The listing builds one solid part. Answer for the finished solid, in the listing's coordinates (mm). Face numbers are marked on the shaded views. Coordinates: 2 decimals unless noted, no trailing zeros. Loops run counter-clockwise (first coordinate to the right, second up) from the corner with the lowest first, then second, coordinate; pieces in that order, holes last. Notation, with made-up numbers: M 57,5.5 L 91,5.5 A15 cw 91,21.5 Z; hole C -19,17 d6. An arc over 180 degrees is marked long. Answer as CSV lines item,"result". Start each with the question number.
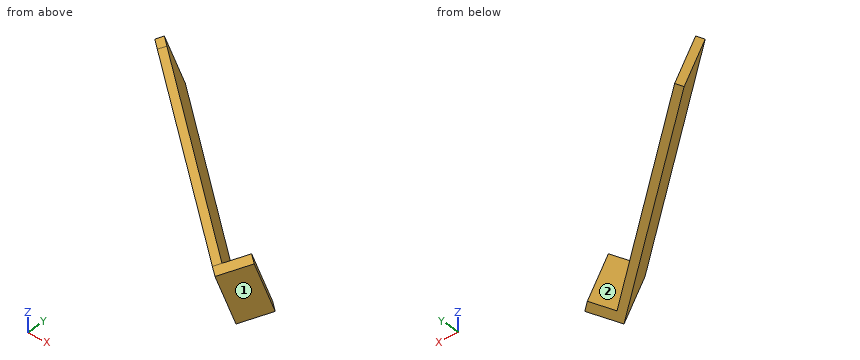
```python
from build123d import *

# Parameters (mm, degrees)
SALIENTE_EXTRUIR1_START = 3.1
SALIENTE_EXTRUIR1_DEPTH = 1
SALIENTE_EXTRUIR2_START = -1
CROQUIS4_W              = 1.301297423
CROQUIS4_H              = 8.40000117
SALIENTE_EXTRUIR2_DEPTH = 4.1


with BuildPart() as part:
    # Croquis3 → Saliente-Extruir1 (new body)
    with BuildSketch(Plane(origin=(-33.880247059, -37.627827516, -15.480136045), x_dir=(-0.768464217, 0.591770514, 0.243455141), z_dir=(-0.639892762, -0.710672931, -0.292371747)).offset(SALIENTE_EXTRUIR1_START)):
        Polygon((-24.387334523, -104.987555147), (-25.688631315, -104.987555147), (-53.688631947, -104.987557356), (-53.688631947, -96.587556289), (-25.688631947, -96.587556289), (-24.387335186, -96.587556289), align=None)
    extrude(amount=SALIENTE_EXTRUIR1_DEPTH)

    # Croquis4 → Saliente-Extruir2 (add)
    with BuildSketch(Plane(origin=(-35.863914621, -39.830913602, -16.38648846), x_dir=(0.768464217, -0.591770514, -0.243455141), z_dir=(0.639892762, 0.710672931, 0.292371747)).offset(SALIENTE_EXTRUIR2_START)):
        with Locations((54.339280659, -100.787556874)):
            Rectangle(CROQUIS4_W, CROQUIS4_H)
    extrude(amount=SALIENTE_EXTRUIR2_DEPTH)


solid = part.part
```
Item 1: For a pull along Z with two mould halves and no side action, classify the marked faces 1 and 2 as pulls with the +Z half, pulls with the -Z half, needs draft (parallel to the pull), parting line crosses it, or undercut.
Item 2: Consider line 1 (Y direction, x = -0.5, z = 62.25); line 2 (Y direction, x = -13.5, z = 68.25); line 3 (X direction, y = -101.75, z = 66.75). Determine where each line is inside the solid, lowest interval first.
Item 3: Each of these flat-tipped pins is pushed along its axis until it touches: P1, Ø4, axis at x = -11, z = 69.5, coming from the +Y side; P2, Ø8, axis at x = -12, y = -98, coming from the +Z side; P3, Ø2, axis at x = 1, z = 72, coming from the +Y side; P4, Ø1.5, axis at x = 1.5, y = -108.5, coming from the +Z side. Where does it stop, or does it pass through?
Item 4: Section B-B on z = 72 is taken. Determine the outline of the cut face in (x, y), then the cut area to 3 significant figures.
Item 5: Section D-D on z = 66 is taken. Determine the outline of the cut face in (x, y).
Item 6: Section A-A on y = -108 is taken. Determine the outline of the cut face in (x, z), then the cut area to 3 significant figures.
Item 7: Section C-C on y = -102 is taken. Determine the outline of the cut face in (x, z).
Results are:
1,face 1,"pulls with the -Z half"
1,face 2,"pulls with the +Z half"
2,line 1,"-105.43 to -104.02"
2,line 2,"-96.19 to -94.79"
2,line 3,"-6.64 to -5.08"
3,P1,"y = -95.57"
3,P2,"z = 74.17"
3,P3,"through"
3,P4,"z = 69.06"
4,outline,"M -17.76,-93.9 L -9.95,-100.94 L -8.38,-100.94 L -17.12,-93.07 Z"
4,area,"11.6 mm²"
5,outline,"M -15.53,-93.44 L 5.75,-112.6 L 8.38,-109.2 L 7.38,-108.3 L 5.39,-110.87 L -13.97,-93.44 Z"
6,outline,"M -0.77,69.09 L 3.38,60.01 L 4.94,60.01 L 0.79,69.09 Z; M 5.71,60.01 L 7.4,60.01 L 8.38,63.09 L 7.38,65.28 Z"
6,area,"21.3 mm²"
7,outline,"M -8.57,71.56 L -4.42,62.48 L -2.85,62.48 L -7,71.56 Z"
